The model under review builds one solid part; all positions refer to its coordinate system, in mm. Give positions to 0.01 mm unless a question says otherwise; leave off trailing zeros. Order: outer loops, then holes, each group sorted by start corner. A loop starts at its lowest first (then second) coordinate and runs counter-clockwise, first axis right, second up.
```python
from build123d import *

# Parameters (mm, degrees)
F0_W     = 12.7
F0_H     = 12.7
F1_DEPTH = 304.8
F3_D     = 6.7564
F4_D     = 5.1054


with BuildPart() as f1:
    # F0 (on Front) → F1 (new body)
    with BuildSketch(Plane.XZ):
        with Locations((6.35, 6.35)):
            Rectangle(F0_W, F0_H)
    extrude(amount=F1_DEPTH)

    # F3 (through all)
    with Locations(Plane.YZ.offset(12.7)):
        with Locations((-228.6, 6.35)):
            Hole(F3_D / 2)

    # F4 (through all)
    with Locations(Plane.YZ.offset(12.7)):
        with Locations((-76.2, 6.35)):
            Hole(F4_D / 2)


solid = f1.part
```
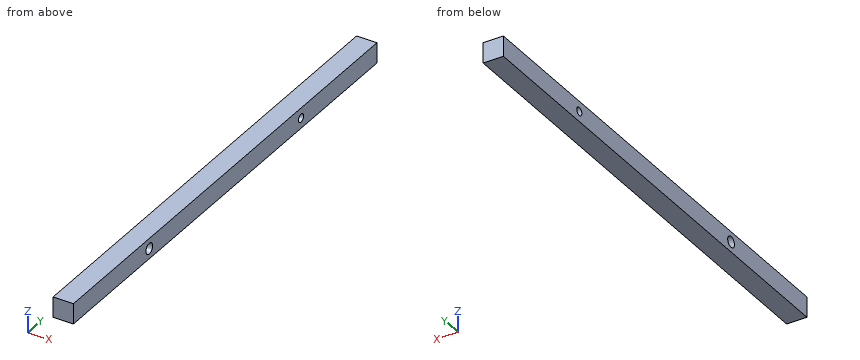
1. Take a section at B-B (y = -76.2). Write out the cut boundary in (x, z).
2. To check wall thickness, follow line 1 (Y direction, x = 1.5, z = 6.75); line 2 (Y direction, x = 3.75, z = 6.25); line 3 (Z direction, x = 7.25, y = -76.2). State the ranges of each line that lie inside material, in increasing order.
3. Take a section at A-A (z = 6.35). Write out the cut boundary in (x, y).
4. Take a section at C-C (y = -228.6). Write out the cut boundary in (x, z).
Answer:
1. outline: (0, 0) - (12.7, 0) - (12.7, 3.8) - (0, 3.8) - close; (0, 8.9) - (12.7, 8.9) - (12.7, 12.7) - (0, 12.7) - close
2. line 1: y = -304.8 to -231.95, -225.25 to -78.72, -73.68 to 0
2. line 2: y = -304.8 to -231.98, -225.22 to -78.75, -73.65 to 0
2. line 3: z = 0 to 3.8, 8.9 to 12.7
3. outline: (0, -304.8) - (12.7, -304.8) - (12.7, -231.98) - (0, -231.98) - close; (0, -225.22) - (12.7, -225.22) - (12.7, -78.75) - (0, -78.75) - close; (0, -73.65) - (12.7, -73.65) - (12.7, 0) - (0, 0) - close
4. outline: (0, 0) - (12.7, 0) - (12.7, 2.97) - (0, 2.97) - close; (0, 9.73) - (12.7, 9.73) - (12.7, 12.7) - (0, 12.7) - close
